from build123d import *

# Parameters (mm, degrees)
BOSS_EXTRUDE1_DEPTH       = 19.05
M4X0_7_TAPPED_HOLE1_D     = 3.3
M4X0_7_TAPPED_HOLE1_DEPTH = 6.35
M2X0_4_TAPPED_HOLE1_D     = 1.6
M2X0_4_TAPPED_HOLE1_DEPTH = 19.05
FILLET1_R                 = 2.54


with BuildPart() as part:
    # Sketch1 → Boss-Extrude1 (new body)
    with BuildSketch(Plane.XY):
        Polygon((0, 0), (12.7, 0), (12.7, -3.429), (0, -3.429), (0, -6.604), (31.75, -6.604), (31.75, 18.796), (12.7, 18.796), (12.7, 6.35), (0, 6.35), align=None)
    extrude(amount=BOSS_EXTRUDE1_DEPTH)

    # M4x0.7 Tapped Hole1
    with Locations(Plane(origin=(0, 6.35, 0), x_dir=(1, 0, 0), z_dir=(0, 1, 0))):
        with Locations((6.35, -9.525)):
            Hole(M4X0_7_TAPPED_HOLE1_D / 2, depth=M4X0_7_TAPPED_HOLE1_DEPTH)

    # M2x0.4 Tapped Hole1
    with Locations(Plane.XY.offset(19.05)):
        with Locations((27.625, 13.296), (27.625, 3.796)):
            Hole(M2X0_4_TAPPED_HOLE1_D / 2, depth=M2X0_4_TAPPED_HOLE1_DEPTH)

    # Fillet1
    fillet1_edges = [part.edges().sort_by_distance(p)[0] for p in [
        (0, 6.35, 9.525),
        (12.7, 18.796, 9.525),
        (31.75, 18.796, 9.525),
        (31.75, -6.604, 9.525),
        (0, -3.429, 9.525),
        (0, 0, 9.525),
    ]]
    fillet(fillet1_edges, radius=FILLET1_R)


solid = part.part
Geometry check sheet. Reference: the model listing, model coordinates, mm. A direction names the side the tool comes from. Give positions to 0.01 mm unless a question says otherwise; leave off trailing zeros. Write each loop counter-clockwise with the first axis right and the second up, starting at its lowest first coordinate (ties: lowest second). Pieces come first, ordered by that corner, then holes.
1) Cross-section at A-A (x = 4). Record the boundary of the cut face in (y, z), plus the area to 3 significant figures.
Values follow:
outline: (-6.6, 0) - (-3.43, 0) - (-3.43, 19.05) - (-6.6, 19.05) - close; (0, 0) - (6.35, 0) - (6.35, 19.05) - (0, 19.05) - close
area: 181 mm2
2) Thickness scan on line 1 (Y direction, x = 12, z = 4); line 2 (Z direction, x = 6.35, y = 4.25) (3 decimals); line 3 (X direction, y = 4.5, z = 8.5). Record the ranges inside material, lowest first.
Values follow:
line 1: y = -6.6 to -3.43, 0 to 6.35
line 2: z = 0 to 7.875, 11.175 to 19.05
line 3: x = 0.1 to 5.06, 7.64 to 27.25, 28 to 31.75
3) Cross-section at B-B (x = 7.5). Record the boundary of the cut face in (y, z), plus the area to 3 significant figures.
Values follow:
outline: (-6.6, 0) - (-3.43, 0) - (-3.43, 19.05) - (-6.6, 19.05) - close; (0, 0) - (6.35, 0) - (6.35, 8.34) - (0, 8.34) - close; (0, 10.71) - (6.35, 10.71) - (6.35, 19.05) - (0, 19.05) - close
area: 166 mm2
4) Cross-section at C-C (z = 17.5). Record the boundary of the cut face in (x, y) (3 decimals).
Values follow:
outline: (0, -6.604) - (29.21, -6.604) arc R2.54 ccw to (31.75, -4.064) - (31.75, 16.256) arc R2.54 ccw to (29.21, 18.796) - (15.24, 18.796) arc R2.54 ccw to (12.7, 16.256) - (12.7, 6.35) - (2.54, 6.35) arc R2.54 ccw to (0, 3.81) - (0, 2.54) arc R2.54 ccw to (2.54, 0) - (12.7, 0) - (12.7, -3.429) - (2.54, -3.429) arc R2.54 ccw to (0, -5.969) - close; hole circle Ø1.6 at (27.625, 3.796); hole circle Ø1.6 at (27.625, 13.296)
5) Cross-section at D-D (y = 7.25). Record the boundary of the cut face in (x, z).
Values follow:
outline: (12.7, 0) - (31.75, 0) - (31.75, 19.05) - (12.7, 19.05) - close
6) Set-up check for faces 1 (the face through (26.862, 4.036, 9.392)), 2 (the face through (30.986, -5.88, 9.658)), 3 (the face through (12.7, 11, 9)), 4 (the face through (8, -3.429, 9)), 5 (the face through (5.59, 3.13, 10.99)): record each of +Z, -Z, +X, -X, +Y, -Y from which the full face is reachable in a straight line by a thin tool's end or side.
Values follow:
face 1: +Z, -Z
face 2: +Z, -Z, +X, -Y
face 3: +Z, -Z, -X, +Y
face 4: +Z, -Z, -X
face 5: +Y
7) Release check for a two-part mould opening along Y. For faces 6 (the face through (9, 6.35, 9)), 7 (the face through (19, 6, 19.05)), 8 (the face through (0.764, 0.724, 9.658)), 9 (the face through (14, -6.604, 9)) record: released by +Y, released by -Y, zero draft, split by the parting line, or undercut.
Values follow:
face 6: released by +Y
face 7: zero draft
face 8: undercut
face 9: released by -Y
8) Go/stop test with flat-tipped pins: pin 1 Ø1 at (x, y) = (27.625, 13.296) entering from +Z; pin 2 Ø1 at (y, z) = (-1.5, 8) entering from -X; pin 3 Ø6 at (x, z) = (6, 11.5) entering from +Y. Record where each tip stops, or that it passes through.
Values follow:
pin 1: passes through
pin 2: stops at x = 12.7
pin 3: stops at y = 6.35
